Study the drawing (mm; zero at the part's minimum x, y, z) and answer. A direction names the side the tool comes from. Coordinates: 2 decimals unless noted, no trailing zeros. Write each loop counter-clockwise with the first axis right and the second up, starting at its lowest first coordinate (ties: lowest second). Pieces come first, ordered by that corner, then holes. Notation, with made-up numbers: M 42,2 L 57,2 A14 cw 57,6 Z; hole C -24.75,74.5 d5. An arc over 180 degrees is marked long. Answer as a JSON object with one key per item and string values. Group by question number.
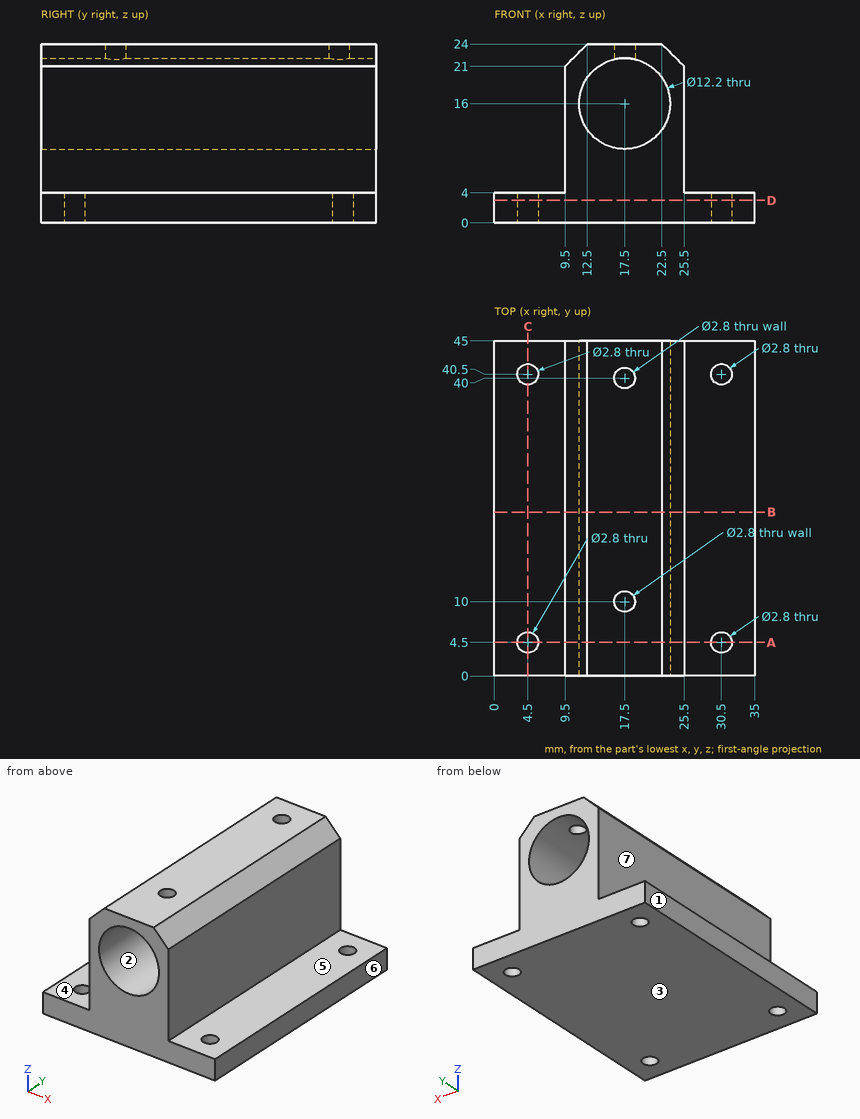
Item 1: A tool of negligible diameter and unlimited length cuts with its end or side. For the marked faces 5, 6 and 7, from which of +Z, -Z, +X, -X, +Y, -Y can it reach the whole face along a straight path? Write none if from no direction.
Item 2: A cutting plane is placed at B-B, the plane y = 22. Write down the section's boundary in (x, z), and give its area (3 significant figures).
Item 3: A cutting plane is placed at D-D, the plane z = 3. Write down the section's boundary in (x, y).
Item 4: Consider L1, parallel to Y at x = 17.5, z = 22.8; L2, parallel to Y at x = 30.5, z = 2.8; L3, parallel to X at y = 9, z = 16. Determine where each line is inside the solid, lowest interval first. Write a range as from..to.
Item 5: A cutting plane is placed at A-A, the plane y = 4.5. Write down the section's boundary in (x, z), and give its area (3 significant figures).
Item 6: A cutting plane is placed at C-C, the plane x = 4.5. Write down the section's boundary in (y, z), and give its area (3 significant figures).
Item 7: For a pull along Z with two mould halves and no side action, classify the marked faces 1, 2, 3 and 4 as +Z half, -Z half, draft (parallel to the pull), parting line (faces both ways), or undercut.
Item 8: Flat-ended cylindrical pins translate along their axes: pin 1 Ø3.5 at (x, y) = (4.5, 4.5) entering from +Z; pin 2 Ø5 at (y, z) = (24, 16.5) entering from -X; pin 3 Ø3.5 at (x, y) = (17.5, 40) entering from -Z; pin 4 Ø5 at (y, z) = (23, 14) entering from +X. Find the tip coordinate at first contact, or state that the pin passes through.
Answer:
{
 "1": {"face 5": "+Z, +X, +Y, -Y", "face 6": "+Z, -Z, +X, +Y, -Y", "face 7": "+Z, -X, +Y, -Y"},
 "2": {"outline": "M 0,0 L 35,0 L 35,4 L 25.5,4 L 25.5,21 L 22.5,24 L 12.5,24 L 9.5,21 L 9.5,4 L 0,4 Z; hole C 17.5,16 d12.2", "area": "334 mm2"},
 "3": {"outline": "M 0,0 L 35,0 L 35,45 L 0,45 Z; hole C 4.5,4.5 d2.8; hole C 4.5,40.5 d2.8; hole C 30.5,4.5 d2.8; hole C 30.5,40.5 d2.8"},
 "4": {"L1": "0..8.6, 11.4..38.6, 41.4..45", "L2": "0..3.1, 5.9..39.1, 41.9..45", "L3": "9.5..11.4, 23.6..25.5"},
 "5": {"outline": "M 0,0 L 3.1,0 L 3.1,4 L 0,4 Z; M 5.9,0 L 29.1,0 L 29.1,4 L 25.5,4 L 25.5,21 L 22.5,24 L 12.5,24 L 9.5,21 L 9.5,4 L 5.9,4 Z; M 31.9,0 L 35,0 L 35,4 L 31.9,4 Z; hole C 17.5,16 d12.2", "area": "312 mm2"},
 "6": {"outline": "M 0,0 L 3.1,0 L 3.1,4 L 0,4 Z; M 5.9,0 L 39.1,0 L 39.1,4 L 5.9,4 Z; M 41.9,0 L 45,0 L 45,4 L 41.9,4 Z", "area": "158 mm2"},
 "7": {"face 1": "draft", "face 2": "undercut", "face 3": "-Z half", "face 4": "+Z half"},
 "8": {"pin 1": "z = 4", "pin 2": "x = 9.5", "pin 3": "z = 0", "pin 4": "x = 25.5"}
}
